Geometry check sheet. Reference: the model listing, model coordinates, mm. Coordinates: 2 decimals unless noted, no trailing zeros. Write each loop counter-clockwise with the first axis right and the second up, starting at its lowest first coordinate (ties: lowest second). Pieces come first, ordered by that corner, then holes. Notation, with made-up numbers: M 30,-19.75 L 64,-19.75 A31 ccw 64,15.25 Z; hole C 32,38 d11. An arc over 180 degrees is marked long. Answer as a JSON object with one key per item and string values. Group by question number.
```python
from build123d import *

# Parameters (mm, degrees)
F_0181_EXTRUDE_DEPTH        = 2.4
F_0181_EXTRUDE_ROTATE_ANGLE = 120
F_0180_REVOLVE_ROTATE_ANGLE = 90
F_0183_CYLINDER_SKETCH_R    = 1.4
F_0183_CYLINDER_DEPTH       = 10


with BuildPart() as part:
    # 0181_extrude_Sketch → 0181_extrude (new body)
    with BuildSketch(Plane.XY):
        Polygon((0, 0), (3.175426481, 0), (4.763139721, 2.75), (3.175426481, 5.5), (0, 5.5), (-1.58771324, 2.75), align=None)
    extrude(amount=F_0181_EXTRUDE_DEPTH)


with BuildPart() as part_1:
    # 0181_extrude_Rotate: moved
    add(part.part.rotate(Axis((0, 0, 0), (0, 0, 1)), F_0181_EXTRUDE_ROTATE_ANGLE))


with BuildPart() as part_2:
    # 0181_extrude_Translate: moved
    add(part_1.part.moved(Location((3.175426481, 0, 0))))


with BuildPart() as body_2:
    # 0180_revolve_Sketch → 0180_revolve (revolve)
    with BuildSketch(Plane.XY, mode=Mode.PRIVATE) as f_0180_revolve_sk:
        Polygon((0, 0), (2.6125, 0), (3.675426481, 0.61368089), (3.675426481, 1.78631911), (2.6125, 2.4), (0, 2.4), align=None)
    revolve(f_0180_revolve_sk.sketch.rotate(Axis((0, -100, 0), (0, 1, 0)), 90), axis=Axis((0, -100, 0), (0, 1, 0)))


with BuildPart() as body_2_1:
    # 0180_revolve_Rotate: moved
    add(body_2.part.rotate(Axis((0, 0, 0), (1, 0, 0)), F_0180_REVOLVE_ROTATE_ANGLE))


with BuildPart() as part_3:
    add(part_2.part)

    # 0182_common: intersect body 2
    add(body_2_1.part, mode=Mode.INTERSECT)


with BuildPart() as body_2_2:
    # 0183_cylinder_Sketch → 0183_cylinder (new body)
    with BuildSketch(Plane.XY):
        Circle(F_0183_CYLINDER_SKETCH_R)
    extrude(amount=F_0183_CYLINDER_DEPTH)


with BuildPart() as body_2_2_1:
    # 0183_cylinder_Translate: moved
    add(body_2_2.part.moved(Location((0, 0, -5))))


with BuildPart() as part_4:
    add(part_3.part)

    # 0184_sub: cut body 2 2
    add(body_2_2_1.part, mode=Mode.SUBTRACT)


solid = part_4.part
```
1) Go/stop test with a flat-tipped pin: pin 1 Ø2 at (x, y) = (2, -2) entering from +Z. Record where the tip stops, or that it passes through.
2) Draft check along Y on faces 1 (the cylindrical face through (-1.4, 0.06, 1.18)), 2 (the flat face through (1.1, -1.1, 0)), 3 (the flat face through (0, -2.75, 1)), 4 (the flat face through (-2.37, 1.394, 1.184)). Enter one of: +Y half, -Y half, draft (parallel to the pull), parting line (faces both ways), or undercut.
3) Section check A-A (z = 1.5). Record the cut outline in (x, y).
4) Material ranges on probe 1 along Y at (x, z) = (-1, 0.5); probe 2 along X at (y, z) = (0.1, 1.3); probe 3 along X at (y, z) = (-0.8, 1.45), recorded low to high. Write a range as [from, to].
Entries:
{
 "1": {"pin 1": "z = 2.4"},
 "2": {"face 1": "undercut", "face 2": "draft", "face 3": "-Y half", "face 4": "+Y half"},
 "3": {"outline": "M -3.18,0 L -1.59,-2.75 L 1.59,-2.75 L 3.18,0 L 1.59,2.75 L -1.59,2.75 Z; hole C 0,0 d2.8"},
 "4": {"probe 1": "[-2.75, -0.98], [0.98, 2.75]", "probe 2": "[-3.12, -1.4], [1.4, 3.12]", "probe 3": "[-2.71, -1.15], [1.15, 2.71]"}
}
